from build123d import *

# Parameters (mm, degrees)
F0_W         = 77
F0_H         = 70
F1_DEPTH     = 8
F2_T         = -2.5
F4_DEPTH     = 13.5
F6_DEPTH     = 2.5
F7_T1_DEPTH  = 82.5
F7_T3_DEPTH  = 46
F7_T5_DEPTH  = 46
F7_T7_DEPTH  = 33.25
F7_T9_DEPTH  = 33.25
F7_T11_DEPTH = 61.25
F7_T13_DEPTH = 11.25
F7_T16_ANGLE = 95.9416658211
F7_T18_ANGLE = 95.9416658211
F7_T23_DEPTH = 39.5
F7_T27_DEPTH = 67.5
F7_T34_DEPTH = 67.5
F7_T38_DEPTH = 39.5


# Not quite as in the source:
# - a fillet or chamfer that OpenCascade refuses, or shapes differently, is made with other operations: its cross-section is extruded or revolved along the edge and cut away or added


with BuildPart() as f1:
    # F0 (on Front) → F1 (new body, symmetric)
    with BuildSketch(Plane.XZ):
        Rectangle(F0_W, F0_H)
    extrude(amount=F1_DEPTH, both=True)

    # F2
    f2_openings = [f1.faces().sort_by_distance(p)[0] for p in [
        (0, 0, 35),
    ]]
    offset(amount=F2_T, openings=f2_openings)

    # F3 (on face) → F4 (cut, through all)
    with BuildSketch(Plane.XZ.offset(8)):
        Polygon((34.5, 35), (-34.5, 35), (-34.5, -20), (-7.5, -20), (7.5, -20), (34.5, -20), align=None)
        with BuildLine():
            Line((7.5, -20), (-7.5, -20))
            Line((-7.5, -20), (-7.5, -25))
            ThreePointArc((-7.5, -25), (-6.8465319688, -28.0618621785), (-5, -30.5901699437))
            ThreePointArc((-5, -30.5901699437), (0, -32.5), (5, -30.5901699437))
            ThreePointArc((5, -30.5901699437), (6.8465319688, -28.0618621785), (7.5, -25))
            Line((7.5, -25), (7.5, -20))
        make_face()
        with BuildLine():
            Line((-5, -30.5901699437), (-5, -35))
            Line((-5, -35), (5, -35))
            Line((5, -35), (5, -30.5901699437))
            ThreePointArc((5, -30.5901699437), (0, -32.5), (-5, -30.5901699437))
        make_face()
    extrude(amount=-F4_DEPTH, mode=Mode.SUBTRACT)

    # F5 (on face) → F6 (cut, through all)
    with BuildSketch(Plane(origin=(0, 8, 0), x_dir=(-1, 0, 0), z_dir=(0, 1, 0))):
        with BuildLine():
            ThreePointArc((2, -2.75), (4.75, 0), (2, 2.75))
            Line((2, 2.75), (-2, 2.75))
            ThreePointArc((-2, 2.75), (-4.75, 0), (-2, -2.75))
            Line((-2, -2.75), (2, -2.75))
        make_face()
    extrude(amount=-F6_DEPTH, mode=Mode.SUBTRACT)

    # F7: fillet of radius 2.5 on 10 edges, made by hand

    # F7_s2 → F7_t1 (cut)
    with BuildSketch(Plane.XY.offset(-41.25)):
        with BuildLine():
            ThreePointArc((38.5, -5.5), (37.767766953, -7.267766953), (36, -8))
            Line((36, -8), (38.5, -8))
            Line((38.5, -8), (38.5, -5.5))
        make_face()
        with BuildLine():
            ThreePointArc((-38.5, -5.5), (-37.767766953, -7.267766953), (-36, -8))
            Line((-36, -8), (-38.5, -8))
            Line((-38.5, -8), (-38.5, -5.5))
        make_face()
    extrude(amount=F7_T1_DEPTH, mode=Mode.SUBTRACT)

    # F7_s4 → F7_t3 (cut)
    with BuildSketch(Plane.YZ.offset(-44.75)):
        with BuildLine():
            ThreePointArc((-5.5, -35), (-7.267766953, -34.267766953), (-8, -32.5))
            Line((-8, -32.5), (-8, -35))
            Line((-8, -35), (-5.5, -35))
        make_face()
    extrude(amount=F7_T3_DEPTH, mode=Mode.SUBTRACT)

    # F7_s6 → F7_t5 (cut)
    with BuildSketch(Plane.YZ.offset(-1.25)):
        with BuildLine():
            ThreePointArc((-8, -32.5), (-7.267766953, -34.267766953), (-5.5, -35))
            Line((-5.5, -35), (-8, -35))
            Line((-8, -35), (-8, -32.5))
        make_face()
    extrude(amount=F7_T5_DEPTH, mode=Mode.SUBTRACT)

    # F7_s8 → F7_t7 (cut)
    with BuildSketch(Plane.YZ.offset(1.25)):
        with BuildLine():
            ThreePointArc((-8, -22.5), (-7.267766953, -20.732233047), (-5.5, -20))
            Line((-5.5, -20), (-8, -20))
            Line((-8, -20), (-8, -22.5))
        make_face()
    extrude(amount=F7_T7_DEPTH, mode=Mode.SUBTRACT)

    # F7_s10 → F7_t9 (cut)
    with BuildSketch(Plane.YZ.offset(-34.5)):
        with BuildLine():
            ThreePointArc((-8, -22.5), (-7.267766953, -20.732233047), (-5.5, -20))
            Line((-5.5, -20), (-8, -20))
            Line((-8, -20), (-8, -22.5))
        make_face()
    extrude(amount=F7_T9_DEPTH, mode=Mode.SUBTRACT)

    # F7_s12 → F7_t11 (cut)
    with BuildSketch(Plane.XY.offset(-20)):
        with BuildLine():
            ThreePointArc((37, -8), (35.232233047, -7.267766953), (34.5, -5.5))
            Line((34.5, -5.5), (34.5, -8))
            Line((34.5, -8), (37, -8))
        make_face()
        with BuildLine():
            ThreePointArc((-37, -8), (-35.232233047, -7.267766953), (-34.5, -5.5))
            Line((-34.5, -5.5), (-34.5, -8))
            Line((-34.5, -8), (-37, -8))
        make_face()
    extrude(amount=F7_T11_DEPTH, mode=Mode.SUBTRACT)

    # F7_s14 → F7_t13 (cut)
    with BuildSketch(Plane.XY.offset(-25)):
        with BuildLine():
            ThreePointArc((10, -8), (8.232233047, -7.267766953), (7.5, -5.5))
            Line((7.5, -5.5), (7.5, -8))
            Line((7.5, -8), (10, -8))
        make_face()
        with BuildLine():
            ThreePointArc((-10, -8), (-8.232233047, -7.267766953), (-7.5, -5.5))
            Line((-7.5, -5.5), (-7.5, -8))
            Line((-7.5, -8), (-10, -8))
        make_face()
    extrude(amount=F7_T13_DEPTH, mode=Mode.SUBTRACT)

    # F7_s15 → F7_t16 (revolve, cut)
    with BuildSketch(Plane.XY.offset(-25)):
        with BuildLine():
            ThreePointArc((-10, -8), (-8.232233047, -7.267766953), (-7.5, -5.5))
            Line((-7.5, -5.5), (-7.5, -8))
            Line((-7.5, -8), (-10, -8))
        make_face()
    revolve(axis=Axis((0, -8, -25), (0, -1, 0)), revolution_arc=F7_T16_ANGLE, mode=Mode.SUBTRACT)

    # F7_s17 → F7_t18 (revolve, cut)
    with BuildSketch(Plane(origin=(2.5739938884, 0, -0.2678883482), x_dir=(0, 1, 0), z_dir=(-0.9946278028, 0, 0.1035158632))):
        with BuildLine():
            ThreePointArc((-8, 34.8656950696), (-7.267766953, 33.0979281167), (-5.5, 32.3656950696))
            Line((-5.5, 32.3656950696), (-8, 32.3656950696))
            Line((-8, 32.3656950696), (-8, 34.8656950696))
        make_face()
    revolve(axis=Axis((0, -8, -25), (0, -1, 0)), revolution_arc=F7_T18_ANGLE, mode=Mode.SUBTRACT)


with BuildPart() as f7_tool21:
    # F7_s22 → F7_t23 (new body)
    with BuildSketch(Plane.YZ.offset(1.25)):
        with BuildLine():
            ThreePointArc((-8, -22.5), (-7.267766953, -20.732233047), (-5.5, -20))
            Line((-5.5, -20), (-8, -20))
            Line((-8, -20), (-8, -22.5))
        make_face()
    extrude(amount=F7_T23_DEPTH)

    split(bisect_by=Plane.YZ.offset(34.5), keep=Keep.TOP)


with BuildPart() as f7_tool25:
    # F7_s26 → F7_t27 (new body)
    with BuildSketch(Plane.XY.offset(-26.25)):
        with BuildLine():
            ThreePointArc((37, -8), (35.232233047, -7.267766953), (34.5, -5.5))
            Line((34.5, -5.5), (34.5, -8))
            Line((34.5, -8), (37, -8))
        make_face()
    extrude(amount=F7_T27_DEPTH)

    split(bisect_by=Plane.XY.offset(-20), keep=Keep.BOTTOM)


with BuildPart() as f7_tool21_1:
    add(f7_tool21.part)

    # F7_t29: intersect F7_tool25
    add(f7_tool25.part, mode=Mode.INTERSECT)


with BuildPart() as f1_1:
    add(f1.part)

    # F7_t19: cut F7_tool21
    add(f7_tool21_1.part, mode=Mode.SUBTRACT)


with BuildPart() as f7_tool32:
    # F7_s33 → F7_t34 (new body)
    with BuildSketch(Plane.XY.offset(41.25)):
        with BuildLine():
            ThreePointArc((-37, -8), (-35.232233047, -7.267766953), (-34.5, -5.5))
            Line((-34.5, -5.5), (-34.5, -8))
            Line((-34.5, -8), (-37, -8))
        make_face()
    extrude(amount=-F7_T34_DEPTH)

    split(bisect_by=Plane.XY.offset(-20), keep=Keep.BOTTOM)


with BuildPart() as f7_tool36:
    # F7_s37 → F7_t38 (new body)
    with BuildSketch(Plane.YZ.offset(-40.75)):
        with BuildLine():
            ThreePointArc((-8, -22.5), (-7.267766953, -20.732233047), (-5.5, -20))
            Line((-5.5, -20), (-8, -20))
            Line((-8, -20), (-8, -22.5))
        make_face()
    extrude(amount=F7_T38_DEPTH)

    split(bisect_by=Plane.YZ.offset(-34.5), keep=Keep.BOTTOM)


with BuildPart() as f7_tool32_1:
    add(f7_tool32.part)

    # F7_t40: intersect F7_tool36
    add(f7_tool36.part, mode=Mode.INTERSECT)


with BuildPart() as f1_2:
    add(f1_1.part)

    # F7_t30: cut F7_tool32
    add(f7_tool32_1.part, mode=Mode.SUBTRACT)


solid = f1_2.part
Source: CAD feature listing. Evaluate the final solid. Frame: model axes, mm. A direction names the side the tool comes from. Coordinates: 2 decimals unless noted, no trailing zeros. Loops run counter-clockwise (first coordinate to the right, second up) from the corner with the lowest first, then second, coordinate; pieces in that order, holes last. Notation, with made-up numbers: (30.5, -25.5) -> (80.5, -25.5) arc R15 ccw to (80.5, -5.5) -> close; hole circle Ø6 at (2, -23.5). An arc over 180 degrees is marked (long way). Answer in a Markdown table with one row per item. Add a question column.
Q1. Section A-A on y = -3.5. Return the cut outline in (x, z), and give its area (3 significant figures).
Q2. Section B-B on z = 4. Return the cut outline in (x, y).
Q3. Ray query, line 1 along Y through (x, z) = (18, -24); line 2 along X through (y, z) = (5, 10); line 3 along Z through (x, y) = (32, -4.75). Return the intervals inside material, ascending.
Q4. Section C-C on x = 25. Return the cut outline in (y, z).
Q5. Contact query for flat-ended pins moving along their axis: pin 1 Ø5 at (x, z) = (-3, -4) entering from -Y; pin 2 Ø9 at (x, y) = (-26, 2.5) entering from +Z; pin 3 Ø9 at (x, y) = (13.5, -1.5) entering from +Z. Output: stop coordinate, or through.
Q6. Reachability of faces 1 (the face through (8, -7, -23)), 2 (the face through (-21, 0, -32.5)), 3 (the face through (-4.75, 6.77, -0.06)), 4 (the face through (-21.984, -7.248, -34.287)), 5 (the face through (5, -1, -33)) from +Z, -Z, +X, -X, +Y, -Y: full face, straight path, thin tool, end or side. Return the list, or none.
Q7. Pull-direction query (X, two-part tool) for faces 6 (the face through (35, -7, 6)), 7 (the face through (-38.5, 1, 0)), 8 (the face through (-1, 6, -35)); classes: pulls with the +X half, pulls with the -X half, needs draft (parallel to the pull), parting line crosses it, or undercut.
Computed values:
| question | item | result |
|---|---|---|
| 1 | outline | (-38.5, -35) -> (-5, -35) -> (-5, -32.5) -> (-36, -32.5) -> (-36, 35) -> (-38.5, 35) -> close; (5, -35) -> (38.5, -35) -> (38.5, 35) -> (36, 35) -> (36, -32.5) -> (5, -32.5) -> close |
| 1 | area | 505 mm^2 |
| 2 | outline | (-38.5, -5.5) arc R2.5 ccw to (-36.5, -7.95) arc R2.5 ccw to (-34.5, -5.5) -> (-36, -5.5) -> (-36, 5.5) -> (36, 5.5) -> (36, -5.5) -> (34.5, -5.5) arc R2.5 ccw to (36.5, -7.95) arc R2.5 ccw to (38.5, -5.5) -> (38.5, 8) -> (-38.5, 8) -> close |
| 3 | line 1 | y = -8 to -5.5, 5.5 to 8 |
| 3 | line 2 | x = -38.5 to -36, 36 to 38.5 |
| 3 | line 3 | z = -35 to -32.5 |
| 4 | outline | (-8, -32.5) arc R2.5 ccw to (-5.5, -35) -> (8, -35) -> (8, 35) -> (5.5, 35) -> (5.5, -32.5) -> (-5.5, -32.5) -> (-5.5, -20) arc R2.5 ccw to (-8, -22.5) -> close |
| 5 | pin 1 | stops at y = 5.5 |
| 5 | pin 2 | stops at z = 35 |
| 5 | pin 3 | stops at z = -20 |
| 6 | face 1 | +Z, -Y |
| 6 | face 2 | +Z |
| 6 | face 3 | +Y, -Y |
| 6 | face 4 | -Z, +X, -X, -Y |
| 6 | face 5 | +Z, -Z, -Y |
| 7 | face 6 | undercut |
| 7 | face 7 | pulls with the -X half |
| 7 | face 8 | needs draft |
